from build123d import *

# Parameters (mm, degrees)
F1_DEPTH = 6.35


with BuildPart() as f1:
    # F0 (on Front) → F1 (new body, symmetric)
    with BuildSketch(Plane.XZ):
        with BuildLine():
            Line((-63.5, 25.4), (43.18, 25.4))
            Line((43.18, 25.4), (43.18, 54.975352))
            ThreePointArc((43.18, 54.975352), (48.785666, 72.859274), (63.596736, 84.343627))
            add(Edge.make_bspline(
                [(-63.5, 25.4), (-25.21287, 74.923909), (20.350938, 82.18553), (63.596736, 84.343627)],
                knots=[0, 0, 0, 0, 132.266939, 132.266939, 132.266939, 132.266939], degree=3))
        make_face()
    extrude(amount=F1_DEPTH, both=True)


solid = f1.part
CAD build for the part. Positions are in the model's coordinates, mm. Round coordinates to 2 decimals unless told otherwise and drop trailing zeros. One line per question, with ' | ' between items. Start each with the question number.
Item 1: Wall check: line 1 (Z direction, x = -13.5, y = -4.5); line 2 (Z direction, x = 26.5, y = -4); line 3 (X direction, y = 3.5, z = 54). Give the ranges that are in metal, low to high.
Item 2: Pin check, flat tips, straight feed: pin 1 Ø5 at (x, y) = (-16, 2.5) entering from +Z; pin 2 Ø1.5 at (y, z) = (-4, 61.5) entering from -X; pin 3 Ø1 at (x, y) = (-9.5, 5) entering from +Z. Stop position of each tip, or through.
Item 3: Two-plate mould, pull along Y, no slides. Class faces 1 (the flat face through (-11, 0, 25.4)), 2 (the flat face through (13, -6.35, 49)), 3 (the flat face through (13, 6.35, 49)): pulls with the +Y half, pulls with the -Y half, needs draft (parallel to the pull), parting line crosses it, or undercut.
Responses:
1) line 1: z = 25.4 to 67.51 | line 2: z = 25.4 to 80.44 | line 3: x = -35.16 to 43.18
2) pin 1: stops at z = 67.51 | pin 2: stops at x = -25.5 | pin 3: stops at z = 69.64
3) face 1: needs draft | face 2: pulls with the -Y half | face 3: pulls with the +Y half
